```python
from build123d import *

# Parameters (mm, degrees)
BOSS_EXTRUDE1_DEPTH   = 5.75
BOSS_EXTRUDE1_2_DEPTH = 5.75
BOSS_EXTRUDE2_DEPTH   = 5.75
SKETCH3_R             = 1.75
CUT_EXTRUDE2_DEPTH    = 19.122150851
FILLET1_R             = 2


with BuildPart() as part:
    # Sketch2 → Boss-Extrude1 (new, symmetric)
    with BuildSketch(Plane.XY):
        with BuildLine():
            ThreePointArc((8.364209467, 2), (8.540848945, 1.006925665), (8.6, 0))
            Line((8.6, 0), (16.364209467, 0))
            Line((16.364209467, 0), (16.364209467, 2))
            Line((16.364209467, 2), (8.364209467, 2))
        make_face()
    extrude(amount=BOSS_EXTRUDE1_DEPTH, both=True)



with BuildPart() as body_2:
    # Sketch2 → Boss-Extrude1 2 (new, symmetric)
    with BuildSketch(Plane.XY):
        with BuildLine():
            Line((-16.364209467, 0), (-8.6, 0))
            ThreePointArc((-8.6, 0), (-8.540848945, 1.006925665), (-8.364209467, 2))
            Line((-8.364209467, 2), (-16.364209467, 2))
            Line((-16.364209467, 2), (-16.364209467, 0))
        make_face()
    extrude(amount=BOSS_EXTRUDE1_2_DEPTH, both=True)


with BuildPart() as part_1:
    add(part.part)

    add(body_2.part)  # Boss-Extrude2 merges body 2
    # Sketch2_4 → Boss-Extrude2 (add, symmetric)
    with BuildSketch(Plane.XY):
        with BuildLine():
            Line((8.6, 0), (6.6, 0))
            ThreePointArc((6.6, 0), (5.914302048, 2.929339736), (3.999687488, 5.25))
            Line((3.999687488, 5.25), (-3.999687488, 5.25))
            ThreePointArc((-3.999687488, 5.25), (-5.914302048, 2.929339736), (-6.6, 0))
            Line((-6.6, 0), (-8.6, 0))
            ThreePointArc((-8.6, 0), (-7.541266186, 4.133921179), (-4.625743184, 7.25))
            Line((-4.625743184, 7.25), (4.625743184, 7.25))
            ThreePointArc((4.625743184, 7.25), (7.541266186, 4.133921179), (8.6, 0))
        make_face()
    extrude(amount=BOSS_EXTRUDE2_DEPTH, both=True)

    # Sketch3 → Cut-Extrude2 (cut, through all)
    with BuildSketch(Plane(origin=(0, 2, 0), x_dir=(1, 0, 0), z_dir=(0, 1, 0))):
        with Locations(Location((-10.535, -0.5, 0), (0, 0, 270))):
            Circle(SKETCH3_R)
    cut_extrude2 = extrude(amount=-CUT_EXTRUDE2_DEPTH, mode=Mode.SUBTRACT)

    # Mirror1: Cut-Extrude2 across plane
    add(cut_extrude2.mirror(Plane(origin=(0, 0, 0), x_dir=(0, 0, 1), z_dir=(1, 0, 0))), mode=Mode.SUBTRACT)

    # Fillet1
    fillet1_edges = [part_1.edges().sort_by_distance(p)[0] for p in [
        (16.364209467, 1, 5.75),
        (-16.364209467, 1, 5.75),
        (-16.364209467, 1, -5.75),
        (16.364209467, 1, -5.75),
    ]]
    fillet(fillet1_edges, radius=FILLET1_R)


solid = part_1.part
```
Geometry: final body of the model. Coordinates: model frame, mm. A direction names the side the tool comes from. Coordinates: 2 decimals unless noted, no trailing zeros. Loops run counter-clockwise (first coordinate to the right, second up) from the corner with the lowest first, then second, coordinate; pieces in that order, holes last. Notation, with made-up numbers: M 18.25,87.5 L 24.25,87.5 A19 ccw 24.25,100.5 Z; hole C 89.25,10 d4. An arc over 180 degrees is marked long. Put each result on its own line as item: value.
(1) Cut plane D-D on z = -2. Return the cut outline in (x, y), then the cut area to 3 significant figures.
Answer sheet:
outline: M -16.36,0 L -6.6,0 A6.6 cw -4,5.25 L 4,5.25 A6.6 cw 6.6,0 L 16.36,0 L 16.36,2 L 8.36,2 A8.6 ccw 4.63,7.25 L -4.63,7.25 A8.6 ccw -8.36,2 L -16.36,2 Z
area: 78.0 mm^2
(2) First-contact query: pin 1 (1 mm diameter, centred on x = -10, z = 3, fed in from +Y). Flat tip, straight axial feed; report the tip coordinate or a pass-through.
Answer sheet:
pin 1: stops at y = 2
(3) Material intervals for probe 1 along X at (y, z) = (1.05, 0.5) (3 decimals); probe 2 along X at (y, z) = (1.4, 0.5) (3 decimals); probe 3 along X at (y, z) = (2.25, 0.25), sorted ascending.
Answer sheet:
probe 1: x = -16.364 to -12.285, -8.785 to -6.516, 6.516 to 8.785, 12.285 to 16.364
probe 2: x = -16.364 to -12.285, -8.785 to -6.45, 6.45 to 8.785, 12.285 to 16.364
probe 3: x = -8.3 to -6.2, 6.2 to 8.3
(4) Access query for faces 4 (the face through (0, 5.25, 0)), 5 (the face through (12.4, 2, 0.1)), 6 (the face through (0, 6, 5.75)), 7 (the face through (-16.364, 1, 0)), 8 (the face through (-13, 2, 0)). Directions: +Z, -Z, +X, -X, +Y, -Y. A direction counts if a zero-diameter tool reaches every point of the face in a straight line with its end or side. Return the directions, or none.
Answer sheet:
face 4: +Z, -Z, -Y
face 5: +Z, -Z, +X, +Y
face 6: +Z, +X, -X, +Y, -Y
face 7: +Z, -Z, -X, +Y, -Y
face 8: +Z, -Z, -X, +Y
(5) Draft query along Z for faces 1 (the face through (12.243, 1.014, 0.121)), 2 (the face through (-5.895, 2.967, 0.08)), 3 (the face through (15.76, 1.01, -5.18)). Return one class per face: pulls with the +Z half, pulls with the -Z half, needs draft (parallel to the pull), parting line crosses it, or undercut.
Answer sheet:
face 1: undercut
face 2: needs draft
face 3: pulls with the -Z half
(6) Cut plane B-B on y = 1. Return the cut outline in (x, z) (3 decimals), then the cut area to 3 significant figures.
Answer sheet:
outline: M -16.364,-3.75 A2 ccw -14.364,-5.75 L -6.524,-5.75 L -6.524,5.75 L -14.364,5.75 A2 ccw -16.364,3.75 Z; M 6.524,-5.75 L 14.364,-5.75 A2 ccw 16.364,-3.75 L 16.364,3.75 A2 ccw 14.364,5.75 L 6.524,5.75 Z; hole C -10.535,0.5 d3.5; hole C 10.535,0.5 d3.5
area: 204 mm^2
(7) Cut plane C-C on y = 2.5. Return the cut outline in (x, z).
Answer sheet:
outline: M -8.23,-5.75 L -6.11,-5.75 L -6.11,5.75 L -8.23,5.75 Z; M 6.11,-5.75 L 8.23,-5.75 L 8.23,5.75 L 6.11,5.75 Z
(8) Cut plane A-A on z = 0.5. Return the cut outline in (x, y) (3 decimals).
Answer sheet:
outline: M -16.364,0 L -12.285,0 L -12.285,2 L -16.364,2 Z; M -8.785,0 L -6.6,0 A6.6 cw -4,5.25 L 4,5.25 A6.6 cw 6.6,0 L 8.785,0 L 8.785,2 L 8.364,2 A8.6 ccw 4.626,7.25 L -4.626,7.25 A8.6 ccw -8.364,2 L -8.785,2 Z; M 12.285,0 L 16.364,0 L 16.364,2 L 12.285,2 Z
